The model under review builds one solid part; all positions refer to its coordinate system, in mm. A direction names the side the tool comes from. Round coordinates to 2 decimals unless told otherwise and drop trailing zeros. Order: outer loops, then holes, each group sorted by start corner. A loop starts at its lowest first (then second) coordinate and runs counter-clockwise, first axis right, second up.
Autodesk Inventor part; units mm, degrees
ref_plane "YZ Plane" through (0, 0, 0) normal (1, 0, 0) x (0, 1, 0)
ref_plane "XZ Plane" through (0, 0, 0) normal (0, 1, 0) x (-1, 0, 0)
ref_plane "XY Plane" through (0, 0, 0) normal (0, 0, 1) x (1, 0, 0)
sketch "Эскиз1" plane through (0, 0, 0) normal (0, 0, 1) x (1, 0, 0)
  line L0 (2, -100) -> (-2, -100)
  line L1 (-2, -100) -> (-2, 100)
  line L2 (-2, 100) -> (2, 100)
  line L3 (2, 100) -> (2, -100)
  line L4 (2, -100) -> (-2, 100) construction
  line L5 (-2, -100) -> (2, 100) construction
  point P0 (0, 0)
  dimension "d0" = 4
  dimension "d1" = 200
extrude "Выдавливание1" add sketch "Эскиз1" along normal blind 250
sketch "Эскиз2" plane through (-2, -100, 0) normal (-1, 0, 0) x (0, 0, 1)
  line L0 (250, 200) -> (250, 0)
  line L1 (0, 0) -> (250, 0)
  line L2 (0, 102) -> (250, 102)
  point P0 (0, 100)
sketch "Эскиз3" plane through (2, -100, 0) normal (1, 0, 0) x (0, 0, -1)
  line L0 (0, 0) -> (0, 200) construction
  line L1 (0, 200) -> (-250, 200) construction
  line L2 (-250, 0) -> (-250, 200) construction
  line L3 (0, 0) -> (-250, 0) construction
  line L4 (-250, 200) -> (-250, 0) construction
  line L5 (-250, 0) -> (0, 200) construction
  line L6 (0, 100) -> (-250, 100) construction
  line L7 (0, 200) -> (-250, 200)
  arc A0 (-250, 200) -> (0, 200) centre (-125, 344.0414) ccw
  arc A1 (0, 0) -> (-250, 0) centre (-125, -144.0414) ccw
  line L8 (-250, 0) -> (0, 0)
extrude "Выдавливание2" cut sketch "Эскиз3" against normal blind 4
fillet "Сопряжение1" radius 5 1 edges at (0, 100, 250)
fillet "Сопряжение2" radius 5 1 edges at (0, -100, 250)
sketch "Эскиз4" plane through (-2, -100, 0) normal (-1, 0, 0) x (0, 0, 1)
  arc A0 (250, 189.4287) -> (241.9343, 193.3786) centre (245, 189.4287) ccw
  arc A1 (241.9343, 6.6214) -> (250, 10.5713) centre (245, 10.5713) ccw
  line L0 (248.5, 78.2507) -> (232.9146, 87.249)
  line L1 (230.4146, 91.5791) -> (230.4146, 108.4209)
  line L2 (232.9146, 112.751) -> (248.5, 121.7493)
  arc A2 (232.9146, 112.751) -> (230.4146, 108.4209) centre (235.4146, 108.4209) ccw
  arc A3 (230.4146, 91.5791) -> (232.9146, 87.249) centre (235.4146, 91.5791) ccw
  arc A4 (248.5, 121.7493) -> (250, 124.3473) centre (247, 124.3473) ccw
  arc A5 (250, 75.6527) -> (248.5, 78.2507) centre (247, 75.6527) ccw
  line L3 (250, 124.3473) -> (250, 75.6527)
  line L4 (250, 10.5713) -> (250, 189.4287)
  point P0 (0, 100)
  point P1 (250, 100)
  point P2 (250, 77.3847)
  point P3 (230.4146, 88.6924)
  point P4 (230.4146, 111.3076)
  point P5 (250, 122.6153)
  dimension "d8" = 5
  dimension "d9" = 3
extrude "Выдавливание3" cut sketch "Эскиз4" against normal blind 4
properties part number "грань тела"
(1) Consider section A-A (x = 1.2). Write out the cut boundary in (y, z), and give its area (3 significant figures).
Data:
outline: (-100, 0) - (100, 0) arc R190.72 cw to (93.38, 241.93) arc R5 ccw to (89.43, 250) - (24.35, 250) arc R3 ccw to (21.75, 248.5) - (12.75, 232.91) arc R5 cw to (8.42, 230.41) - (-8.42, 230.41) arc R5 cw to (-12.75, 232.91) - (-21.75, 248.5) arc R3 ccw to (-24.35, 250) - (-89.43, 250) arc R5 ccw to (-93.38, 241.93) arc R190.72 cw to start
area: 33,300 mm2
(2) Consider section B-B (z = 79.5). Write out the cut boundary in (x, y), and give its area (3 significant figures).
Data:
outline: (-2, -58.83) - (2, -58.83) - (2, 58.83) - (-2, 58.83) - close
area: 471 mm2
(3) Consider section C-C (y = -15.5). Write out the cut boundary in (x, z).
Data:
outline: (-2, 0) - (2, 0) - (2, 237.68) - (-2, 237.68) - close
(4) Draft analysis for pull direction Y (two halves, no side actions). For faces 1 (the cylindrical face through (0.028, 53.355, 121.617)), 2 (the flat face through (2, 1, 123)), 3 (the flat face through (-0.03, 17.19, 240.6)), state which applies: pulls with the +Y half, pulls with the -Y half, needs draft (parallel to the pull), parting line crosses it, or undercut.
Data:
face 1: pulls with the +Y half
face 2: needs draft
face 3: undercut
(5) Insertion check: pin 1 (1.2 mm diameter, centred on x = -1, y = 1, fed in from +Z); pin 2 (1.5 mm diameter, centred on x = 0, y = -70, fed in from -Z). Each pin has a flat end and moves straight along its axis. Give the tip position at first contact, or say it passes through.
Data:
pin 1: stops at z = 230.41
pin 2: stops at z = 0
(6) For faces 4 (the cylindrical face through (0.028, 93.953, 247.129)), 5 (the flat face through (-0.028, -17.313, 240.816)), list the 3-axis set-ups (+Z, -Z, +X, -X, +Y, -Y) from which the entire face can be reached by the end or side of a thin tool; tool diameter is ignored.
Data:
face 4: +X, -X, +Y
face 5: +Z, +X, -X
(7) To check wall thickness, follow probe 1 along Z at (x, y) = (0.25, 3); probe 2 along Z at (x, y) = (-1.1, 71); probe 3 along Z at (x, y) = (0.35, -10). State the ranges of each line that lie inside material, in increasing order.
Data:
probe 1: z = 0 to 230.41
probe 2: z = 0 to 44.82, 205.18 to 250
probe 3: z = 0 to 230.67
